Input: part model. Units: mm. Frame: model coordinates. A direction names the side the tool comes from. Round coordinates to 2 decimals unless told otherwise and drop trailing zeros. Order: outer loops, then holes, each group sorted by start corner. A loop starts at its lowest first (then second) coordinate and runs counter-clockwise, first axis right, second up.
Item 1: Cut plane B-B on x = -18. Output: boundary loops of the cut face in (y, z), then the cut area to 3 significant figures.
Item 2: Cut plane A-A on z = -7. Output: boundary loops of the cut face in (x, y), then the cut area to 3 significant figures.
Item 3: Line query: L1, parallel to Z at x = -18, y = 0.75; L2, parallel to Y at x = -12, z = -21; L3, parallel to Y at x = -8, z = -19. Output: solid intervals per line, ascending.
Item 4: Mould query, pull axis X, two halves, no side actions, for faces 6 (the cylindrical face through (-17.792, 0.789, -21.586)), 7 (the flat face through (0, 1, -12)), 8 (the flat face through (-11, -4.9, -24)). Classes: released by +X, released by -X, zero draft, split by the parting line, or undercut.
Item 5: Cut plane C-C on y = 2.25. Output: boundary loops of the cut face in (x, z), then the cut area to 3 significant figures.
Item 6: Reachability of faces 1 (the flat face through (-10, -2, -20)), 2 (the flat face through (-11, 4, -5)), 3 (the flat face through (-4, 1, -23)), 4 (the flat face through (-7.5, 4, -7)), 5 (the flat face through (-11, 6.6, -7)) from +Z, -Z, +X, -X, +Y, -Y: full face, straight path, thin tool, end or side. Return the list, or none.
Item 7: Cut plane D-D on z = -20.5. Output: boundary loops of the cut face in (x, y), then the cut area to 3 significant figures.
Item 8: First-contact query: pin 1 (12 mm diameter, centred on x = -2, z = -8.5, fed in from -Y); pin 2 (4.5 mm diameter, centred on y = 3.5, z = -7, fed in from -X); pin 3 (1.2 mm diameter, centred on y = 5.5, z = -7, fed in from +X); pin 4 (1.3 mm diameter, centred on x = -18, y = 0.5, fed in from -Z). Flat tips, straight axial feed; report the tip coordinate or a pass-through.
Autodesk Inventor part; units mm, degrees
ref_plane "YZ Plane" through (0, 0, 0) normal (1, 0, 0) x (0, 1, 0)
ref_plane "XZ Plane" through (0, 0, 0) normal (0, 1, 0) x (-1, 0, 0)
ref_plane "XY Plane" through (0, 0, 0) normal (0, 0, 1) x (1, 0, 0)
sketch "Эскиз1" plane through (0, 0, 0) normal (0, 1, 0) x (-1, 0, 0)
  line L0 (2, 0) -> (19, 0)
  line L1 (21, -2) -> (21, -21)
  line L2 (19, -23) -> (2, -23)
  line L3 (0, -21) -> (0, -2)
  circle A0 centre (18, -20) radius 1.6
  circle A1 centre (3, -20) radius 1.6
  arc A2 (19, -23) -> (21, -21) centre (19, -21) ccw
  arc A3 (0, -21) -> (2, -23) centre (2, -21) ccw
  arc A4 (2, 0) -> (0, -2) centre (2, -2) ccw
  arc A5 (21, -2) -> (19, 0) centre (19, -2) ccw
  point P0 (0, 0)
  dimension "d6" = 2
  dimension "d20" = 15
  dimension "d21" = 3
  dimension "d22" = 3
extrude "Выдавливание1" add sketch "Эскиз1" along normal blind 1.6
sketch "Эскиз2" plane through (0, 1.6, 0) normal (0, 1, 0) x (1, 0, 0)
  circle A0 centre (-18, 20) radius 1.6
  circle A1 centre (-3, 20) radius 1.6
  line L0 (-10.5, 27.5) -> (-5.5, 27.5)
  line L1 (-5.5, 27.5) -> (-15.5, 27.5)
  line L2 (-15.5, 27.5) -> (-5.5, 27.5)
  line L3 (-5.5, 27.5) -> (-5.5, 20)
  line L4 (-5.5, 20) -> (-15.5, 20)
  line L5 (-15.5, 20) -> (-15.5, 27.5)
  point P0 (0, 0)
extrude "Выдавливание2" add sketch "Эскиз2" against normal blind 6.5 contours L0 L3 L4 L5 L1
sketch "Эскиз3" plane through (0, 1.6, 0) normal (0, 1, 0) x (1, 0, 0)
  line L0 (-5.5, 20) -> (-15.5, 20)
  line L1 (-10.5, 20) -> (-10.5, 5)
  line L2 (-10.5, 5) -> (-13.5, 5)
  line L3 (-10.5, 5) -> (-7.5, 5)
  line L4 (-13.5, 5) -> (-7.5, 5)
  line L5 (-7.5, 5) -> (-7.5, 9)
  line L6 (-7.5, 9) -> (-13.5, 9)
  line L7 (-13.5, 9) -> (-13.5, 5)
  line L8 (-21, 21) -> (-21, 2)
  line L9 (0, 2) -> (0, 21)
  point P0 (0, 0)
  dimension "d14" = 15
  dimension "d15" = 3
  dimension "d16" = 3
  dimension "d17" = 4
  dimension "d23" = 7.5
  dimension "d24" = 7.5
extrude "Выдавливание3" add sketch "Эскиз3" along normal blind 5
properties part number "Temp_Module"
From the geometry:
1. outline: (0, -23) - (1.6, -23) - (1.6, -21.6) - (0, -21.6) - close; (0, -18.4) - (1.6, -18.4) - (1.6, 0) - (0, 0) - close
1. area: 31.7 mm2
2. outline: (-21, 0) - (0, 0) - (0, 1.6) - (-7.5, 1.6) - (-7.5, 6.6) - (-13.5, 6.6) - (-13.5, 1.6) - (-21, 1.6) - close
2. area: 63.6 mm2
3. L1: z = -23 to -21.6, -18.4 to 0
3. L2: y = -4.9 to 1.6
3. L3: y = 0 to 1.6
4. face 6: undercut
4. face 7: released by +X
4. face 8: zero draft
5. outline: (-13.5, -9) - (-7.5, -9) - (-7.5, -5) - (-13.5, -5) - close
5. area: 24.0 mm2
6. face 1: +Z, +X, -X, -Y
6. face 2: +Z, +X, -X, +Y
6. face 3: -Z, +X, +Y, -Y
6. face 4: +Z, -Z, +X, +Y
6. face 5: +Z, -Z, +X, -X, +Y
7. outline: (-21, 0) - (-19.52, 0) - (-19.52, 1.6) - (-21, 1.6) - close; (-16.48, 0) - (-15.5, 0) - (-15.5, -4.9) - (-5.5, -4.9) - (-5.5, 0) - (-4.52, 0) - (-4.52, 1.6) - (-16.48, 1.6) - close; (-1.48, 0) - (0, 0) - (0, 1.6) - (-1.48, 1.6) - close
7. area: 72.9 mm2
8. pin 1: stops at y = 0
8. pin 2: stops at x = -21
8. pin 3: stops at x = -7.5
8. pin 4: stops at z = -23
